Can you work these out from the model? Positions are in its coordinate system, mm. Face numbers are marked on the shaded views. Coordinates: 2 decimals unless noted, no trailing zeros. Loops run counter-clockwise (first coordinate to the right, second up) from the corner with the lowest first, then second, coordinate; pieces in that order, holes last. Notation, with made-up numbers: (33.5, -39.5) -> (46.5, -39.5) arc R34 ccw to (46.5, -8.5) -> close; hole circle Ø2 at (0.25, 20.25). An arc over 180 degrees is marked (long way). Use one line per item in the form item = value. Start each with the question number.
(1) I need wall thicknesses on line 1 (Y direction, x = 2, z = 2); line 2 (Z direction, x = 16.5, y = 19.5). Which ranges of each line are inside material? Lowest first, please. Write a range as [from, to].
(2) Imagine slicing it at C-C (x = 18.5). State how many separate pieces and enclosed holes the cut face has, plus the area to 3 significant figures.
(3) Imagine slicing it at A-A (z = 21). List the corners of the cut face in (x, y) for me, plus the area to 3 significant figures.
(4) Thinking about a two-plate mould opening in Y: for the marked faces 1 and 2, which applies, released by +Y, released by -Y, zero draft, split by the parting line, or undercut?
(5) Imagine slicing it at B-B (y = 21). List the corners of the cut face in (x, z) for me, plus the area to 3 significant figures.
(6) I'm going to push flat-ended pins straight in: pin 1 (2.5 mm diameter, centred on x = 11, z = 32.5, fed in from -Y); pin 2 (6 mm diameter, centred on x = -14.5, z = 34.5, fed in from -Y); pin 3 (8 mm diameter, centred on x = -5, y = -13, fed in from +Z). Where does each tip first touch, or does it pass through?
```python
from build123d import *

# Parameters (mm, degrees)
F0_W     = 50
F0_H     = 23.5
F0_H_2   = 1
F1_DEPTH = 0.6
F2_DEPTH = 50
F4_DEPTH = 50


# Not quite as in the source:
# - a feature names something its author has since deleted; it is built from what else it names


with BuildPart() as f1:
    # F0 (on Top) → F1 (new body)
    with BuildSketch(Plane.XY):
        with Locations((0, 12.25)):
            Rectangle(F0_W, F0_H)
        Polygon((-23.8, 22.1436935786), (-23.8, 22.8), (-22.3194224806, 22.8), (22.3194224806, 22.8), (23.8, 22.8), (23.8, 22.1436935786), (23.8, 2.3563064214), (23.8, 1.7), (22.3194224806, 1.7), (-22.3194224806, 1.7), (-23.8, 1.7), (-23.8, 2.3563064214), align=None, mode=Mode.SUBTRACT)
        with Locations((0, -12.25)):
            Rectangle(F0_W, F0_H)
        Polygon((-22.3194224806, -22.8), (-23.8, -22.8), (-23.8, -22.1436935786), (-23.8, -2.3563064214), (-23.8, -1.7), (-22.3194224806, -1.7), (22.3194224806, -1.7), (23.8, -1.7), (23.8, -2.3563064214), (23.8, -22.1436935786), (23.8, -22.8), (22.3194224806, -22.8), align=None, mode=Mode.SUBTRACT)
        with Locations((0, -24.5)):
            Rectangle(F0_W, F0_H_2)
        Rectangle(F0_W, F0_H_2)
        with Locations((0, 24.5)):
            Rectangle(F0_W, F0_H_2)
        Polygon((-22.3194224806, 22.8), (-23.8, 22.8), (-23.8, 22.1436935786), (-1.4805775194, 12.25), (0, 12.9063064214), align=None)
        Polygon((23.8, 22.8), (22.3194224806, 22.8), (0, 12.9063064214), (1.4805775194, 12.25), (23.8, 22.1436935786), align=None)
        Polygon((1.4805775194, 12.25), (0, 12.9063064214), (-1.4805775194, 12.25), (0, 11.5936935786), align=None)
        Polygon((23.8, 2.3563064214), (1.4805775194, 12.25), (0, 11.5936935786), (22.3194224806, 1.7), (23.8, 1.7), align=None)
        Polygon((-1.4805775194, 12.25), (-23.8, 2.3563064214), (-23.8, 1.7), (-22.3194224806, 1.7), (0, 11.5936935786), align=None)
        Polygon((-23.8, -1.7), (-23.8, -2.3563064214), (-1.4805775194, -12.25), (0, -11.5936935786), (-22.3194224806, -1.7), align=None)
        Polygon((0, -11.5936935786), (-1.4805775194, -12.25), (0, -12.9063064214), (1.4805775194, -12.25), align=None)
        Polygon((22.3194224806, -1.7), (0, -11.5936935786), (1.4805775194, -12.25), (23.8, -2.3563064214), (23.8, -1.7), align=None)
        Polygon((0, -12.9063064214), (22.3194224806, -22.8), (23.8, -22.8), (23.8, -22.1436935786), (1.4805775194, -12.25), align=None)
        Polygon((-23.8, -22.1436935786), (-23.8, -22.8), (-22.3194224806, -22.8), (0, -12.9063064214), (-1.4805775194, -12.25), align=None)
    extrude(amount=-F1_DEPTH)

    # F0 (on Top) → F2 (join)
    with BuildSketch(Plane.XY):
        with Locations((0, 24.5)):
            Rectangle(F0_W, F0_H_2)
        Rectangle(F0_W, F0_H_2)
        with Locations((0, -24.5)):
            Rectangle(F0_W, F0_H_2)
    extrude(amount=F2_DEPTH)

    # F3 (on face) → F4 (join, through all)
    with BuildSketch(Plane(origin=(-25, 0, 0), x_dir=(0, -1, 0), z_dir=(-1, 0, 0))):
        Polygon((-24, 45), (-24, 44.6), (-23.6, 45), align=None)
        Polygon((-24, 40), (-24, 39.6), (-23.6, 40), align=None)
        Polygon((-24, 35), (-24, 34.6), (-23.6, 35), align=None)
        Polygon((-24, 30), (-24, 29.6), (-23.6, 30), align=None)
        Polygon((-24, 25), (-24, 24.6), (-23.6, 25), align=None)
        Polygon((-24, 20), (-24, 19.6), (-23.6, 20), align=None)
        Polygon((-24, 15), (-24, 14.6), (-23.6, 15), align=None)
        Polygon((-24, 10), (-24, 9.6), (-23.6, 10), align=None)
        Polygon((-24, 5), (-24, 4.6), (-23.6, 5), align=None)
        Polygon((0.9, 5), (0.5, 5), (0.5, 4.6), align=None)
        Polygon((0.9, 10), (0.5, 10), (0.5, 9.6), align=None)
        Polygon((0.9, 15), (0.5, 15), (0.5, 14.6), align=None)
        Polygon((0.9, 20), (0.5, 20), (0.5, 19.6), align=None)
        Polygon((0.9, 25), (0.5, 25), (0.5, 24.6), align=None)
        Polygon((0.9, 30), (0.5, 30), (0.5, 29.6), align=None)
        Polygon((0.9, 35), (0.5, 35), (0.5, 34.6), align=None)
        Polygon((0.9, 40), (0.5, 40), (0.5, 39.6), align=None)
        Polygon((0.9, 45), (0.5, 45), (0.5, 44.6), align=None)
        Polygon((25.4, 45), (25, 45), (25, 44.6), align=None)
        Polygon((25.4, 40), (25, 40), (25, 39.6), align=None)
        Polygon((25.4, 35), (25, 35), (25, 34.6), align=None)
        Polygon((25, 30), (25, 29.6), (25.4, 30), align=None)
        Polygon((25, 25), (25, 24.6), (25.4, 25), align=None)
        Polygon((25, 20), (25, 19.6), (25.4, 20), align=None)
        Polygon((25, 15), (25, 14.6), (25.4, 15), align=None)
        Polygon((25, 10), (25, 9.6), (25.4, 10), align=None)
        Polygon((25, 5), (25, 4.6), (25.4, 5), align=None)
    extrude(amount=-F4_DEPTH)


solid = f1.part
```
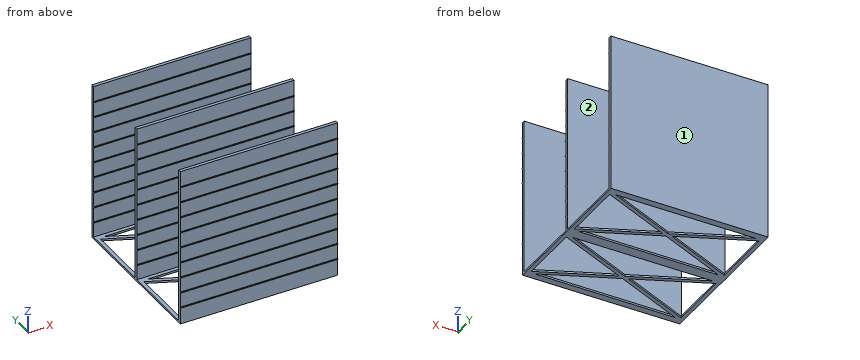
Worked out:
q1.line_1 = [-25, -24], [-0.5, 0.5], [24, 25]
q1.line_2 = [-0.6, 0]
q2.separate_pieces = 7
q2.enclosed_holes = 0
q2.area = 160 mm2
q3.outline = (-25, -25) -> (25, -25) -> (25, -24) -> (-25, -24) -> close; (-25, -0.5) -> (25, -0.5) -> (25, 0.5) -> (-25, 0.5) -> close; (-25, 24) -> (25, 24) -> (25, 25) -> (-25, 25) -> close
q3.area = 150 mm2
q4.face_1 = released by +Y
q4.face_2 = undercut
q5.outline = (-25, -0.6) -> (-23.8, -0.6) -> (-23.8, 0) -> (-25, 0) -> close; (-21.22, -0.6) -> (-18.26, -0.6) -> (-18.26, 0) -> (-21.22, 0) -> close; (18.26, -0.6) -> (21.22, -0.6) -> (21.22, 0) -> (18.26, 0) -> close; (23.8, -0.6) -> (25, -0.6) -> (25, 0) -> (23.8, 0) -> close
q5.area = 4.99 mm2
q6.pin_1 = -25
q6.pin_2 = -25.4
q6.pin_3 = 0
